```python
from build123d import *

# Parameters (mm, degrees)
F0_R     = 2.5
F1_DEPTH = 14.25
F3_D     = 3
F3_DEPTH = 3
F3_TIP   = 0.9012909285
F4_R     = 2.1505871319
F5_DEPTH = 5


with BuildPart() as f1:
    # F0 (on Top) → F1 (new body)
    with BuildSketch(Plane.XY):
        Circle(F0_R)
        with BuildLine():
            ThreePointArc((-1, 1.1180339887), (1.5, 0), (-1, -1.1180339887))
            Line((-1, -1.1180339887), (-1, 1.1180339887))
        make_face(mode=Mode.SUBTRACT)
    extrude(amount=F1_DEPTH)

    # F3
    with Locations(Plane(origin=(0, 0, 0), x_dir=(1, 0, 0), z_dir=(0, 0, -1))):
        with Locations((0, 0)):
            Hole(F3_D / 2, depth=F3_DEPTH)
            with Locations((0, 0, -(F3_DEPTH + F3_TIP / 2))):  # 118° drill point
                Cone(0, F3_D / 2, F3_TIP, mode=Mode.SUBTRACT)

    # F4 (on face) → F5 (join)
    with BuildSketch(Plane.XY.offset(14.25)):
        Circle(F4_R)
        with BuildLine():
            ThreePointArc((-1, 1.1180339887), (1.5, 0), (-1, -1.1180339887))
            Line((-1, -1.1180339887), (-1, 1.1180339887))
        make_face(mode=Mode.SUBTRACT)
        with BuildLine():
            Line((-1, 1.1180339887), (-1, -1.1180339887))
            ThreePointArc((-1, -1.1180339887), (1.5, 0), (-1, 1.1180339887))
        make_face()
    extrude(amount=-F5_DEPTH)


solid = f1.part
```
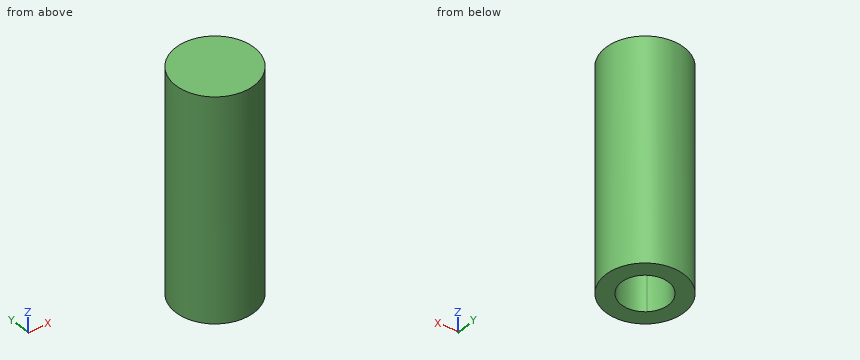
The listing builds one solid part. Answer for the finished solid, in the listing's coordinates (mm). Coordinates: 2 decimals unless noted, no trailing zeros. Write each loop counter-clockwise with the first axis right and the second up, starting at its lowest first coordinate (ties: lowest second). Pieces come first, ordered by that corner, then holes. Notation, with made-up numbers: M 34,4 L 39,4 A10 cw 39,9 Z; hole C -16.5,12.5 d8. An arc over 180 degrees is marked long. Use a Markdown table: item, result. Add a question column.
1. Given P1, Ø1, axis at x = -2, z = 8.5, coming from the +Y side; P2, Ø1.2, axis at x = 0, y = 0, coming from the -Z side, each flat-ended and moving along its own axis, determine where each tip first touches the part or whether it passes through.
2. Section B-B (x = 0) is taken. Give the vertices of the cut face in (y, z), plus the area to 3 significant figures.
3. Section A-A (y = 0) is taken. Give the vertices of the cut face in (x, z), plus the area to 4 significant figures.
4. Straight lines are drawn through the part: line 1 along Y through (x, z) = (0, 6.75); line 2 along Z through (x, y) = (0.35, -0.85); line 3 along X through (y, z) = (0.95, 8.75). For each, find the intervals that lie inside material, in ascending order. Write a range as [from, to].
5. Section C-C (z = 5.25) is taken. Give the vertices of the cut face in (x, y), plus the area to 3 significant figures.
6. Section D-D (z = 12.5) is taken. Give the vertices of the cut face in (x, y), plus the area to 3 significant figures.
Data:
| question | item | result |
|---|---|---|
| 1 | P1 | stops at y = 2 |
| 1 | P2 | stops at z = 9.25 |
| 2 | outline | M -2.5,0 L -1.5,0 L -1.5,9.25 L 1.5,9.25 L 1.5,0 L 2.5,0 L 2.5,14.25 L -2.5,14.25 Z |
| 2 | area | 43.5 mm2 |
| 3 | outline | M -2.5,0 L -1.5,0 L -1.5,3 L -1,3.3 L -1,9.25 L 1.5,9.25 L 1.5,0 L 2.5,0 L 2.5,14.25 L -2.5,14.25 Z |
| 3 | area | 46.55 mm2 |
| 4 | line 1 | y = [-2.5, -1.5], [1.5, 2.5] |
| 4 | line 2 | z = [9.25, 14.25] |
| 4 | line 3 | x = [-2.31, -1], [1.16, 2.31] |
| 5 | outline | C 0,0 d5; hole M -1,-1.12 A1.5 ccw long -1,1.12 Z |
| 5 | area | 13.3 mm2 |
| 6 | outline | C 0,0 d5 |
| 6 | area | 19.6 mm2 |
